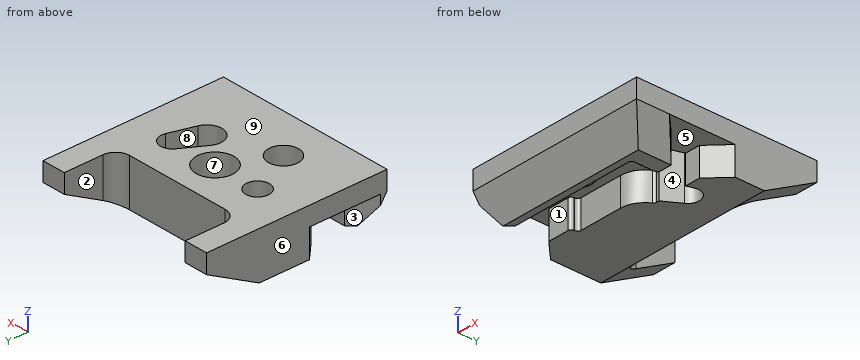
from build123d import *

# Parameters (mm, degrees)
OUTER_FRAME_EXTRUDE_DEPTH      = 5
OUTER_FRAME_EXTRUDE_DEPTH_BACK = 2
OUTSIDE_FRAME_W                = 19.2
OUTSIDE_FRAME_H                = 19.2
OUTSIDE_FRAME_W_2              = 14.2
OUTSIDE_FRAME_H_2              = 14.2
HOTSWAP_BASE_W                 = 19.2
HOTSWAP_BASE_H                 = 13.6
HOTSWAP_BASE_BLOCK_DEPTH       = 5
CUT_EXTRUDE4_DEPTH             = 17.288646353
CUT_EXTRUDE4_DEPTH_BACK        = 17.288646353
SKETCH1_W                      = 2
SKETCH1_H                      = 5.6
CUT_EXTRUDE1_DEPTH             = 4
SWITCH_PIN_HOLES_R             = 2
SWITCH_PIN_HOLES_R_2           = 1.25
SWITCH_HOLES_DEPTH             = 4
HOTSWAP_HOLES_R                = 1.6
CUT_EXTRUDE3_DEPTH             = 17.288646353
CHAMFER1_SIZE                  = 2
BOSS_EXTRUDE2_DEPTH            = 2.5
BOSS_EXTRUDE3_DEPTH            = 2.5
FILLET1_R                      = 0.35
FILLET2_R                      = 1.5
SPLIT1_START                   = -4
SPLIT1_OUTLINE_W               = 19.2
SPLIT1_OUTLINE_H               = 19.2
SPLIT1_OUTLINE_W_2             = 14.2
SPLIT1_OUTLINE_H_2             = 14.2
SPLIT1_DEPTH                   = 5
CHAMFER2_SIZE                  = 2
CHAMFER2_SIZE2                 = 2.998873489


# Read off the part's stored shape, not the designer's step: Split1
with BuildPart() as part:
    # Outside Frame → Outer Frame Extrude (new, two sides: drawn at the far end of the back side and taken through both)
    with BuildSketch(Plane.XY.offset(-4).offset(-OUTER_FRAME_EXTRUDE_DEPTH_BACK)):
        Rectangle(OUTSIDE_FRAME_W, OUTSIDE_FRAME_H)
        Rectangle(OUTSIDE_FRAME_W_2, OUTSIDE_FRAME_H_2, mode=Mode.SUBTRACT)
    extrude(amount=OUTER_FRAME_EXTRUDE_DEPTH + OUTER_FRAME_EXTRUDE_DEPTH_BACK)

    # Hotswap Base → Hotswap Base Block (add)
    with BuildSketch(Plane.XY.offset(-4)):
        with Locations((0, -2.8)):
            Rectangle(HOTSWAP_BASE_W, HOTSWAP_BASE_H)
    extrude(amount=-HOTSWAP_BASE_BLOCK_DEPTH)

    # Sketch1 → Cut-Extrude4 (cut, two sides: drawn at the far end of the back side and taken through both)
    with BuildSketch(Plane(origin=(0, 0, 0), x_dir=(0, 0, -1), z_dir=(1, 0, 0)).offset(-CUT_EXTRUDE4_DEPTH_BACK)):
        with Locations((5, 6.8)):
            Rectangle(SKETCH1_W, SKETCH1_H)
    extrude(amount=CUT_EXTRUDE4_DEPTH + CUT_EXTRUDE4_DEPTH_BACK, mode=Mode.SUBTRACT)

    # Hotswap Well → Cut-Extrude1 (cut)
    with BuildSketch(Plane(origin=(0, 0, -6), x_dir=(-1, 0, 0), z_dir=(0, 0, -1))):
        with BuildLine():
            Line((-10, -1.1), (-2.355843798, -1.1))
            ThreePointArc((-2.355843798, -1.1), (-1.396424004, -2.19317122), (0, -2.6))
            Line((0, -2.6), (5, -2.6))
            Line((5, -2.6), (5, -3.35))
            Line((5, -3.35), (10, -3.35))
            Line((10, -3.35), (10, -6.9))
            Line((10, -6.9), (-6, -6.9))
            Line((-6, -6.9), (-6, -4.1))
            Line((-6, -4.1), (-10, -4.1))
            Line((-10, -4.1), (-10, -1.1))
        make_face()
    extrude(amount=CUT_EXTRUDE1_DEPTH, mode=Mode.SUBTRACT)

    # Switch Pin Holes → Switch Holes (cut)
    with BuildSketch(Plane.XY.offset(-4)):
        Circle(SWITCH_PIN_HOLES_R)
        with Locations((-5, 0)):
            Circle(SWITCH_PIN_HOLES_R_2)
        with Locations((5, 0)):
            Circle(SWITCH_PIN_HOLES_R_2)
    extrude(amount=-SWITCH_HOLES_DEPTH, mode=Mode.SUBTRACT)

    # Hotswap Holes → Cut-Extrude3 (cut, through all)
    with BuildSketch(Plane.XY):
        with Locations((-2.560136595, -4.965291588)):
            Circle(HOTSWAP_HOLES_R)
        with BuildLine():
            Line((3.930924016, 0.647747281), (2.46548889, -1.77088348))
            ThreePointArc((2.46548889, -1.77088348), (3.179147124, -4.059894044), (5.3631684, -3.070485887))
            Line((5.3631684, -3.070485887), (6.194736133, -0.367567099))
            ThreePointArc((6.194736133, -0.367567099), (5.511530489, 1.140542222), (3.930924016, 0.647747281))
        make_face()
    extrude(amount=-CUT_EXTRUDE3_DEPTH, mode=Mode.SUBTRACT)

    # Chamfer1
    chamfer1_edges = [part.edges().sort_by_distance(p)[0] for p in [
        (9.6, -4.1, -7.5),
        (-9.6, -6.9, -7.5),
        (-9.6, -3.35, -7.5),
        (9.6, -1.1, -7.5),
    ]]
    chamfer(chamfer1_edges, length=CHAMFER1_SIZE)

    # Sketch2 → Boss-Extrude2 (add)
    with BuildSketch(Plane(origin=(9.6, 0, 0), x_dir=(0, 0, -1), z_dir=(1, 0, 0))):
        Polygon((6, 9.6), (9, 4), (4, 4), (4, 9.6), align=None)
    extrude(amount=-BOSS_EXTRUDE2_DEPTH)

    # Sketch3 → Boss-Extrude3 (add)
    with BuildSketch(Plane.ZY.offset(9.6)):
        Polygon((-4, 9.6), (-6, 9.6), (-9, 4), (-4, 4), align=None)
    extrude(amount=-BOSS_EXTRUDE3_DEPTH)

    # Fillet1
    fillet1_edges = [part.edges().sort_by_distance(p)[0] for p in [
        (6, -4.1, -7.5),
        (-5, -3.35, -7.5),
        (-5, -2.6, -7.5),
        (6, -6.9, -7.5),
        (2.355843798, -1.1, -7.5),
    ]]
    fillet(fillet1_edges, radius=FILLET1_R)

    # Fillet2
    fillet2_edges = [part.edges().sort_by_distance(p)[0] for p in [
        (7.1, 4, -6.5),
        (-7.1, 4, -6.5),
    ]]
    fillet(fillet2_edges, radius=FILLET2_R)

    # Split1 outline → Split1 (cut)
    with BuildSketch(Plane.XY.offset(SPLIT1_START)):
        Rectangle(SPLIT1_OUTLINE_W, SPLIT1_OUTLINE_H)
        Rectangle(SPLIT1_OUTLINE_W_2, SPLIT1_OUTLINE_H_2, mode=Mode.SUBTRACT)
    extrude(amount=SPLIT1_DEPTH, mode=Mode.SUBTRACT)

    # Chamfer2
    chamfer2_edges = [part.edges().sort_by_distance(p)[0] for p in [
        (9.6, -7.85, -9),
        (0, -9.6, -9),
    ]]
    chamfer2_side = [part.faces().sort_by_distance(p)[0] for p in [
        (1.357387596, -7.916485347, -9),
    ]]
    chamfer(chamfer2_edges, length=CHAMFER2_SIZE, length2=CHAMFER2_SIZE2, reference=chamfer2_side[0])


solid = part.part
Verification items for the finished model (mm, model axes). Face numbers are marked on the shaded views. A direction names the side the tool comes from. Coordinates: 2 decimals unless noted, no trailing zeros. Order: outer loops, then holes, each group sorted by start corner. A loop starts at its lowest first (then second) coordinate and runs counter-clockwise, first axis right, second up. Notation, with made-up numbers: M 64.25,-26 L 94.25,-26 A20 cw 94.25,-18 Z; hole C 78,19.25 d8. An arc over 180 degrees is marked long. One line per item, written item: value. Start each with the question number.
Item 1: Sectioned sample at D-D (y = 1.75). Enter the section's corners in (x, z).
Item 2: Access from +Z, -Z, +X, -X, +Y, -Y to the whole of each face (thin tool, end or side, straight path). Record for the marked faces 1, 2, 3, 4 and 5.
Item 3: Scan lines: probe 1 along Y at (x, z) = (0, -6.15); probe 2 along X at (y, z) = (7.75, -6.2); probe 3 along Y at (x, z) = (-4, -4.9). Record each from-to range of solid material in increasing order.
Item 4: Sectioned sample at B-B (y = -5.25). Enter the section's corners in (x, z).
Item 5: Sectioned sample at A-A (x = -3.5). Enter the section's corners in (y, z).
Item 6: Mould release check, pull along X, two halves, no side actions. Record for the marked faces 6, 7, 8 and 9: released by +X, released by -X, zero draft, split by the parting line, or undercut.
Item 7: Gauge pin test, flat ends, axial feed: pin 1 (3 mm diameter, centred on x = 3.83, y = -2.6, fed in from -Z); pin 2 (0.6 mm diameter, centred on x = 7, z = -7, fed in from +Y); pin 3 (0.9 mm diameter, centred on x = -0.5, z = -7.5, fed in from +Y); pin 4 (2 mm diameter, centred on x = 4, z = -8, fed in from -Y). Record the tip position at first contact, or that the pin passes through.
Item 8: Sectioned sample at C-C (x = 1). Enter the section's corners in (y, z).
Conclusion:
1. outline: M -9.6,-9 L 9.6,-9 L 9.6,-4 L 0.97,-4 L 0.97,-8 L -0.97,-8 L -0.97,-4 L -9.6,-4 Z
2. face 1: -Z, +X, -X
2. face 2: +Z, -Z, +Y
2. face 3: -Z, -X
2. face 4: +Z, -Z
2. face 5: -Z
3. probe 1: y = -9.5 to -6.9, -2.6 to -2, 2 to 4
3. probe 2: x = -9.6 to -7.1, 7.1 to 9.6
3. probe 3: y = -9.6 to -5.66, -4.27 to -0.75, 0.75 to 4
4. outline: M -9.6,-6 L -4.13,-6 L -4.13,-4 L -9.6,-4 Z; M -0.99,-6 L 6,-6 L 6,-9 L 7.6,-9 L 8.75,-7.28 L 8.75,-6 L 9.6,-6 L 9.6,-4 L -0.99,-4 Z
5. outline: M -9.6,-6 L -7.6,-9 L -6.9,-9 L -6.9,-6 L -6.26,-6 L -6.26,-4 L -9.6,-4 Z; M -3.67,-6 L -2.6,-6 L -2.6,-9 L 4,-9 L 4,-4 L -3.67,-4 Z
6. face 6: released by -X
6. face 7: undercut
6. face 8: undercut
6. face 9: zero draft
7. pin 1: passes through
7. pin 2: stops at y = 8.26
7. pin 3: stops at y = 4
7. pin 4: stops at y = -8.93
8. outline: M -9.6,-6 L -7.6,-9 L -6.9,-9 L -6.9,-6 L -2.4,-6 L -2.4,-9 L 4,-9 L 4,-4 L 1.73,-4 L 1.73,-8 L -1.73,-8 L -1.73,-4 L -9.6,-4 Z
